from build123d import *

# Parameters (mm, degrees)
SKETCH1_W           = 50.8
SKETCH1_H           = 50.8
BOSS_EXTRUDE1_DEPTH = 25.4
SKETCH2_W           = 5.08
SKETCH2_H           = 5.08
CUT_EXTRUDE1_DEPTH  = 84.007883963
FILLET1_R           = 2.54
SKETCH3_W           = 5.08
SKETCH3_H           = 7.62
BOSS_EXTRUDE2_DEPTH = 25.4
FILLET2_R           = 2.54
CUT_EXTRUDE2_DEPTH  = 79.288057838


with BuildPart() as part:
    # Sketch1 → Boss-Extrude1 (new body)
    with BuildSketch(Plane.XY):
        with BuildLine():
            Line((0, 55.88), (50.8, 55.88))
            ThreePointArc((50.8, 55.88), (54.392102448, 54.392102448), (55.88, 50.8))
            Line((55.88, 50.8), (55.88, -2.54))
            ThreePointArc((55.88, -2.54), (54.392102448, -6.132102448), (50.8, -7.62))
            Line((50.8, -7.62), (0, -7.62))
            ThreePointArc((0, -7.62), (-3.592102448, -6.132102448), (-5.08, -2.54))
            Line((-5.08, -2.54), (-5.08, 50.8))
            ThreePointArc((-5.08, 50.8), (-3.592102448, 54.392102448), (0, 55.88))
        make_face()
        with Locations((25.4, 25.4)):
            Rectangle(SKETCH1_W, SKETCH1_H, mode=Mode.SUBTRACT)
    extrude(amount=BOSS_EXTRUDE1_DEPTH)

    # Sketch2 → Cut-Extrude1 (cut, through all)
    with BuildSketch(Plane.XY.offset(25.4)):
        with Locations((25.4, 53.34)):
            Rectangle(SKETCH2_W, SKETCH2_H)
    extrude(amount=-CUT_EXTRUDE1_DEPTH, mode=Mode.SUBTRACT)

    # Fillet1
    fillet1_edges = [part.edges().sort_by_distance(p)[0] for p in [
        (22.86, 50.8, 12.7),
        (27.94, 50.8, 12.7),
    ]]
    fillet(fillet1_edges, radius=FILLET1_R)

    # Sketch3 → Boss-Extrude2 (add)
    with BuildSketch(Plane.XY.offset(25.4)):
        with Locations((20.32, 59.69)):
            Rectangle(SKETCH3_W, SKETCH3_H)
        with Locations((30.48, 59.69)):
            Rectangle(SKETCH3_W, SKETCH3_H)
    extrude(amount=-BOSS_EXTRUDE2_DEPTH)

    # Fillet2
    fillet2_edges = [part.edges().sort_by_distance(p)[0] for p in [
        (17.78, 55.88, 12.7),
        (17.78, 63.5, 12.7),
        (33.02, 63.5, 12.7),
        (33.02, 55.88, 12.7),
    ]]
    fillet(fillet2_edges, radius=FILLET2_R)

    # Sketch4 → Cut-Extrude2 (cut, through all)
    with BuildSketch(Plane.ZY.offset(-17.78)):
        with BuildLine():
            Line((2.8575, 60.96), (6.0325, 60.96))
            ThreePointArc((6.0325, 60.96), (7.3025, 59.69), (6.0325, 58.42))
            Line((6.0325, 58.42), (2.8575, 58.42))
            ThreePointArc((2.8575, 58.42), (1.5875, 59.69), (2.8575, 60.96))
        make_face()
        with BuildLine():
            Line((11.1125, 60.96), (14.2875, 60.96))
            ThreePointArc((14.2875, 60.96), (15.5575, 59.69), (14.2875, 58.42))
            Line((14.2875, 58.42), (11.1125, 58.42))
            ThreePointArc((11.1125, 58.42), (9.8425, 59.69), (11.1125, 60.96))
        make_face()
        with BuildLine():
            Line((19.3675, 60.96), (22.5425, 60.96))
            ThreePointArc((22.5425, 60.96), (23.8125, 59.69), (22.5425, 58.42))
            Line((22.5425, 58.42), (19.3675, 58.42))
            ThreePointArc((19.3675, 58.42), (18.0975, 59.69), (19.3675, 60.96))
        make_face()
    extrude(amount=-CUT_EXTRUDE2_DEPTH, mode=Mode.SUBTRACT)


solid = part.part
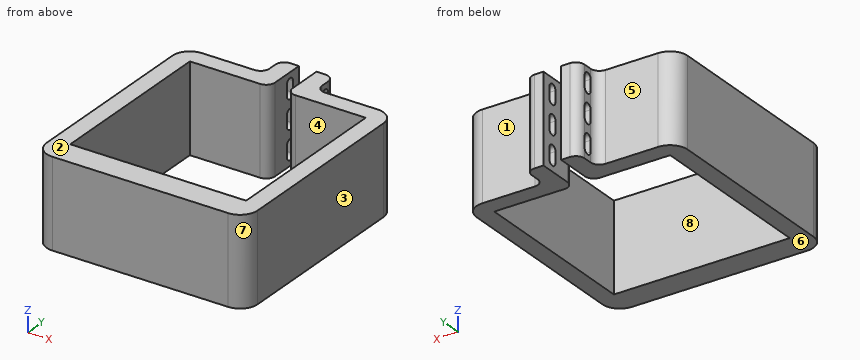
Here's how the part is built. I have some questions about the finished solid (model axes, mm). Face numbers are marked on the shaded views. A direction names the side the tool comes from. Give positions to 0.01 mm unless a question says otherwise; leave off trailing zeros. Order: outer loops, then holes, each group sorted by start corner. A loop starts at its lowest first (then second) coordinate and runs counter-clockwise, first axis right, second up. Notation, with made-up numbers: M -16.75,40.5 L 17.25,40.5 A25 ccw 17.25,63.5 Z; hole C 79.25,24.5 d5. An arc over 180 degrees is marked long. Answer as a JSON object with one key per item and string values. Group by question number.
1) Please list where these lines run through material, in increasing order: L1, parallel to X at y = 23, z = 19.25; L2, parallel to Y at x = 15, z = 22; L3, parallel to Z at x = 21, y = 60.5. Write a range as [from, to].
2) I'm going to push flat-ended pins straight in: pin 1 Ø3 at (y, z) = (59.5, 24.5) entering from -X; pin 2 Ø5 at (y, z) = (61, 12.5) entering from +X; pin 3 Ø4.5 at (x, z) = (10, 17) entering from +Y; pin 4 Ø10 at (x, y) = (15, 42) entering from -Z. Where does each tip first touch, or does it pass through?
3) Suppose I cut it at D-D, the plane y = 9.5. Write out the boundary of the cut face in (x, z), plus the area to 3 significant figures.
4) On a 3-axis mill with a long thin cutter (end or side, diameter ignored), from which of +Z, -Z, +X, -X, +Y, -Y can I reach the whole of each face in a straight line? I mean the marked faces 1, 2, 3, 4 and 5. Say none if no direction works.
5) Suppose I cut it at B-B, the plane x = 42. Write out the boundary of the cut face in (y, z), plus the area to 3 significant figures.
6) Suppose I cut it at A-A, the plane y = 59.69. Count the separate pieces of the cut face and the enclosed holes in it, plus the area to 3 significant figures.
7) We'd pull the mould along X, two halves only. Please class the marked faces 6, 7 and 8: pulls with the +X half, pulls with the -X half, needs draft (parallel to the pull), parting line crosses it, or undercut.
Results found:
{
 "1": {"L1": "[-5.08, 0], [50.8, 55.88]", "L2": "[-7.62, 0], [50.8, 55.88]", "L3": "[0, 1.88], [7.01, 10.13], [15.27, 18.39], [23.52, 25.4]"},
 "2": {"pin 1": "x = 17.75", "pin 2": "x = 33.02", "pin 3": "y = 55.88", "pin 4": "through"},
 "3": {"outline": "M -5.08,0 L 0,0 L 0,25.4 L -5.08,25.4 Z; M 50.8,0 L 55.88,0 L 55.88,25.4 L 50.8,25.4 Z", "area": "258 mm²"},
 "4": {"face 1": "+Z, -Z, +X, +Y", "face 2": "+Z, +X, -X, +Y, -Y", "face 3": "+Z, -Z, +X, +Y, -Y", "face 4": "+Z, -Z", "face 5": "+Z, -Z, -X, +Y"},
 "5": {"outline": "M -7.62,0 L 0,0 L 0,25.4 L -7.62,25.4 Z; M 50.8,0 L 55.88,0 L 55.88,25.4 L 50.8,25.4 Z", "area": "323 mm²"},
 "6": {"separate pieces": "8", "enclosed holes": "0", "area": "83.9 mm²"},
 "7": {"face 6": "needs draft", "face 7": "pulls with the +X half", "face 8": "undercut"}
}
